```python
from build123d import *

# Parameters (mm, degrees)
SKETCH2_R            = 1.5
SKETCH2_R_2          = 1.6
BOSS_EXTRUDE2_DEPTH  = 4.25
SKETCH4_R            = 2.5
HOLES_TO_DRILL_DEPTH = 416.108494854


with BuildPart() as part:
    # Sketch2 → Boss-Extrude2 (new body)
    with BuildSketch(Plane(origin=(0, 0, 0), x_dir=(1, 0, 0), z_dir=(0, 1, 0))):
        Polygon((184.400116, 296), (225.400116, 255), (241.514718626, 255), (282.514718626, 296), (287.485169777, 296), (291, 292.485169777), (291, 287.514718626), (253, 249.514718626), (253, 226.666961), (291, 188.666961), (291, 181.333039), (253, 143.333039), (253, 120.485281374), (291, 82.485281374), (291, 77.514830223), (287.485169777, 74), (282.514718626, 74), (241.514718626, 115), (225.400116, 115), (184.400116, 74), (175.599884, 74), (134.599884, 115), (113.485281374, 115), (72.485281374, 74), (67.514830223, 74), (64, 77.514830223), (64, 82.485281374), (91, 109.485281374), (91, 123), (81.5, 132.5), (81.5, 163.760895), (64, 181.260895), (64, 188.739105), (81.5, 206.239105), (81.5, 237.5), (91, 247), (91, 260.514718626), (64, 287.514718626), (64, 292.485169777), (67.514830223, 296), (72.485281374, 296), (113.485281374, 255), (134.599884, 255), (175.599884, 296), align=None)
        with Locations(Location((180, 80, 0), (0, 0, 270))):
            Circle(SKETCH2_R, mode=Mode.SUBTRACT)
        with Locations(Location((180, 290, 0), (0, 0, 270))):
            Circle(SKETCH2_R, mode=Mode.SUBTRACT)
        with Locations(Location((285, 80, 0), (0, 0, 270))):
            Circle(SKETCH2_R, mode=Mode.SUBTRACT)
        with Locations(Location((70, 290, 0), (0, 0, 270))):
            Circle(SKETCH2_R, mode=Mode.SUBTRACT)
        with Locations(Location((285, 290, 0), (0, 0, 270))):
            Circle(SKETCH2_R, mode=Mode.SUBTRACT)
        with Locations(Location((70, 185, 0), (0, 0, 270))):
            Circle(SKETCH2_R, mode=Mode.SUBTRACT)
        with Locations(Location((180, 185, 0), (0, 0, 270))):
            Circle(SKETCH2_R, mode=Mode.SUBTRACT)
        with Locations(Location((285, 185, 0), (0, 0, 270))):
            Circle(SKETCH2_R, mode=Mode.SUBTRACT)
        with Locations(Location((256.5, 185, 0), (0, 0, 270))):
            Circle(SKETCH2_R_2, mode=Mode.SUBTRACT)
        with Locations(Location((276.5, 185, 0), (0, 0, 270))):
            Circle(SKETCH2_R_2, mode=Mode.SUBTRACT)
        with Locations(Location((106.5, 220, 0), (0, 0, 270))):
            Circle(SKETCH2_R_2, mode=Mode.SUBTRACT)
        with Locations(Location((106.5, 150, 0), (0, 0, 270))):
            Circle(SKETCH2_R_2, mode=Mode.SUBTRACT)
        with Locations(Location((86.5, 220, 0), (0, 0, 270))):
            Circle(SKETCH2_R_2, mode=Mode.SUBTRACT)
        with Locations(Location((86.5, 150, 0), (0, 0, 270))):
            Circle(SKETCH2_R_2, mode=Mode.SUBTRACT)
        with Locations(Location((70, 80, 0), (0, 0, 270))):
            Circle(SKETCH2_R, mode=Mode.SUBTRACT)
        with Locations(Location((181.5, 165.5, 0), (0, 0, 270))):
            Circle(SKETCH2_R, mode=Mode.SUBTRACT)
        with Locations(Location((181.5, 204.5, 0), (0, 0, 270))):
            Circle(SKETCH2_R, mode=Mode.SUBTRACT)
        Polygon((162, 177.02296782), (141.97703218, 157), (124.999970007, 157), (101.5, 180.5), (101.5, 189.5), (124.999970007, 213), (141.97703218, 213), (162, 192.97703218), align=None, mode=Mode.SUBTRACT)
        Polygon((251.5, 210.014709), (240.98529, 220.529449), (224.014709, 220.529449), (197, 193.51474), (197, 176.48526), (224.014709, 149.470551), (240.98529, 149.470551), (251.5, 159.985291), align=None, mode=Mode.SUBTRACT)
        Polygon((143, 246.415771), (143, 229.566314), (159.566314, 213), (199.51474, 213), (216, 229.48526), (216, 247.429580116), (183.682617, 279.746963116), (176.317383, 279.733154), align=None, mode=Mode.SUBTRACT)
        Polygon((143, 123.584229), (143, 140.433686), (159.566314, 157), (199.51474, 157), (216, 140.51474), (216, 122.570419884), (183.682617, 90.253036884), (176.317383, 90.266846), align=None, mode=Mode.SUBTRACT)
        with BuildLine():
            Line((101.500000013, 226.75), (101.500000013, 213.25))
            Line((101.500000013, 213.25), (102.000000013, 212.75))
            Line((102.000000013, 212.75), (102.100000157, 212.75))
            ThreePointArc((102.100000157, 212.75), (105.1, 209.75), (102.100000157, 206.75))
            Line((102.100000157, 206.75), (90.899999843, 206.75))
            ThreePointArc((90.899999843, 206.75), (87.9, 209.75), (90.899999843, 212.75))
            Line((90.899999843, 212.75), (90.999999987, 212.75))
            Line((90.999999987, 212.75), (91.499999987, 213.25))
            Line((91.499999987, 213.25), (91.499999987, 226.75))
            Line((91.499999987, 226.75), (90.999999987, 227.25))
            Line((90.999999987, 227.25), (90.899999843, 227.25))
            ThreePointArc((90.899999843, 227.25), (87.9, 230.25), (90.899999843, 233.25))
            Line((90.899999843, 233.25), (102.100000157, 233.25))
            ThreePointArc((102.100000157, 233.25), (105.100000157, 230.25), (102.100000157, 227.25))
            Line((102.100000157, 227.25), (102.000000013, 227.25))
            Line((102.000000013, 227.25), (101.500000013, 226.75))
        make_face(mode=Mode.SUBTRACT)
        with BuildLine():
            Line((271.500000013, 191.75), (271.500000013, 178.25))
            Line((271.500000013, 178.25), (272.000000013, 177.75))
            Line((272.000000013, 177.75), (272.100000157, 177.75))
            ThreePointArc((272.100000157, 177.75), (275.100000157, 174.75), (272.100000157, 171.75))
            Line((272.100000157, 171.75), (260.899999843, 171.75))
            ThreePointArc((260.899999843, 171.75), (257.9, 174.75), (260.899999843, 177.75))
            Line((260.899999843, 177.75), (260.999999987, 177.75))
            Line((260.999999987, 177.75), (261.499999987, 178.25))
            Line((261.499999987, 178.25), (261.499999987, 191.75))
            Line((261.499999987, 191.75), (260.999999987, 192.25))
            Line((260.999999987, 192.25), (260.899999843, 192.25))
            ThreePointArc((260.899999843, 192.25), (257.9, 195.25), (260.899999843, 198.25))
            Line((260.899999843, 198.25), (272.100000157, 198.25))
            ThreePointArc((272.100000157, 198.25), (275.100000157, 195.25), (272.100000157, 192.25))
            Line((272.100000157, 192.25), (272.000000013, 192.25))
            Line((272.000000013, 192.25), (271.500000013, 191.75))
        make_face(mode=Mode.SUBTRACT)
        with BuildLine():
            Line((101.500000013, 156.75), (101.500000013, 143.25))
            Line((101.500000013, 143.25), (102.000000013, 142.75))
            Line((102.000000013, 142.75), (102.100000157, 142.75))
            ThreePointArc((102.100000157, 142.75), (105.1, 139.75), (102.100000157, 136.75))
            Line((102.100000157, 136.75), (90.899999843, 136.75))
            ThreePointArc((90.899999843, 136.75), (87.9, 139.75), (90.899999843, 142.75))
            Line((90.899999843, 142.75), (90.999999987, 142.75))
            Line((90.999999987, 142.75), (91.499999987, 143.25))
            Line((91.499999987, 143.25), (91.499999987, 156.75))
            Line((91.499999987, 156.75), (90.999999987, 157.25))
            Line((90.999999987, 157.25), (90.899999843, 157.25))
            ThreePointArc((90.899999843, 157.25), (87.9, 160.25), (90.899999843, 163.25))
            Line((90.899999843, 163.25), (102.100000157, 163.25))
            ThreePointArc((102.100000157, 163.25), (105.100000157, 160.25), (102.100000157, 157.25))
            Line((102.100000157, 157.25), (102.000000013, 157.25))
            Line((102.000000013, 157.25), (101.500000013, 156.75))
        make_face(mode=Mode.SUBTRACT)
    extrude(amount=BOSS_EXTRUDE2_DEPTH)

    # Sketch4 → Holes-to-drill (cut, through all)
    with BuildSketch(Plane(origin=(0, 4.25, 0), x_dir=(1, 0, 0), z_dir=(0, 1, 0))):
        with Locations(Location((80.606601718, 279.393398282, 0), (0, 0, 270))):
            Circle(SKETCH4_R)
        with Locations(Location((274.393398282, 279.393398282, 0), (0, 0, 270))):
            Circle(SKETCH4_R)
        with Locations(Location((80.606601718, 90.606601718, 0), (0, 0, 270))):
            Circle(SKETCH4_R)
        with Locations(Location((274.393398282, 90.606601718, 0), (0, 0, 270))):
            Circle(SKETCH4_R)
    extrude(amount=-HOLES_TO_DRILL_DEPTH, mode=Mode.SUBTRACT)


solid = part.part
```
Geometry: final body of the model. Coordinates: model frame, mm. A direction names the side the tool comes from. Round coordinates to 2 decimals unless told otherwise and drop trailing zeros. Use one line per item in the form item = value.
(1) First-contact query: pin 1 Ø3.5 at (x, z) = (86.5, -150) entering from +Y; pin 2 Ø2 at (y, z) = (3.5, -145.5) entering from +X; pin 3 Ø1.3 at (y, z) = (2.5, -251) entering from -X; pin 4 Ø3 at (x, z) = (86.5, -220) entering from +Y. Flat tips, straight axial feed; report the tip coordinate or a pass-through.
Results list:
pin_1 = 4.25
pin_2 = 256.17
pin_3 = 91
pin_4 = through
(2) Section A-A on y = 0.8. Count the separate pieces of the cut face and the enclosed holes in it, and give its area (3 significant figures).
Results list:
separate_pieces = 1
enclosed_holes = 28
area = 19,000 mm^2
(3) Ray query, probe 1 along Z at (x, y) = (234, 2.8); probe 2 along Z at (x, y) = (104, 2.65); probe 3 along Z at (x, y) = (157.5, 2.9). Return the intervals inside material, ascending. Write a range as [from, to].
Results list:
probe_1 = [-255, -220.53], [-149.47, -115]
probe_2 = [-264.49, -232.57], [-227.93, -212.07], [-207.43, -192], [-178, -162.57], [-157.93, -142.07], [-137.43, -105.51]
probe_3 = [-277.9, -260.92], [-215.07, -197.48], [-172.52, -154.93], [-109.08, -92.1]
(4) Access query for faces 4 (the face through (271.734, 2.095, -207.933)), 5 (the face through (200.07, 2.1, -106.64)), 6 (the face through (204.6, 2.1, -275.8)), 7 (the face through (86, 2, -128)). Directions: +Z, -Z, +X, -X, +Y, -Y. A direction counts if a zero-diameter tool reaches every point of the face in a straight line with its end or side. Return the directions, or none.
Results list:
face_4 = +X, +Y, -Y
face_5 = +Y, -Y
face_6 = -Z, +Y, -Y
face_7 = -X, +Y, -Y
(5) Draft query along X for faces 1 (the face through (77.689, 2.095, -273.826)), 2 (the face through (272.266, 2.095, -162.599)), 3 (the face through (152.129, 2.095, -167.152)). Return one class per face: pulls with the +X half, pulls with the -X half, needs draft (parallel to the pull), parting line crosses it, or undercut.
Results list:
face_1 = pulls with the -X half
face_2 = pulls with the +X half
face_3 = undercut
